Part model, mm, in its own coordinate system. Face numbers are marked on the shaded views. A direction names the side the tool comes from. Round coordinates to 2 decimals unless told otherwise and drop trailing zeros. Order: outer loops, then holes, each group sorted by start corner. A loop starts at its lowest first (then second) coordinate and runs counter-clockwise, first axis right, second up. Notation, with made-up numbers: M -33,2.25 L 25,2.25 A26 cw 25,38.25 Z; hole C 8.5,35.25 d9. An arc over 180 degrees is marked long. Write each question's results on one line, items separated by ' | '. Start each with the question number.
1. Two-plate mould, pull along Y, no slides. Class the marked faces 3, 4 and 5: +Y half, -Y half, draft (parallel to the pull), parting line (faces both ways), or undercut.
2. Drop flat-ended pins along their axis: pin 1 Ø1.6 at (x, z) = (45, -8.5) entering from -Y; pin 2 Ø4 at (y, z) = (7.5, 36) entering from -X; pin 3 Ø4 at (x, y) = (38.5, -9.5) entering from +Z. Give the stop position or say it passes through.
3. Probe L1, parallel to Y at x = 5, z = 38; L2, parallel to X at y = 2.25, z = -20; L3, parallel to Z at x = 25, y = 9.5. List the from-to ranges inside material, lowest first. Write a range as [from, to].
4. Band-saw the part on C-C, the plane y = -3.5. List the corners of the cut face in (x, z).
5. Band-saw the part on B-B, the plane y = 1.25. List the corners of the cut face in (x, z), then the cut area to 3 significant figures.
6. Which spindle directions (+Z, -Z, +X, -X, +Y, -Y) get a long thin tool onto all of the face, cutting with end or side? Do the marked faces 1 and 2. Say none if no direction does.
7. Band-saw the part on A-A, the plane z = 29.5. List the corners of the cut face in (x, y).
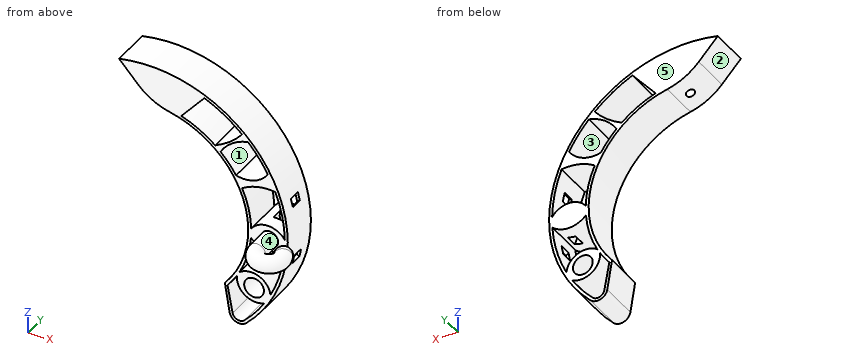
```python
from build123d import *

# Parameters (mm, degrees)
BOSS_EXTRUDE1_DEPTH        = 13.33
FILLET1_R                  = 20
SKETCH3_R                  = 3.33
CUT_EXTRUDE2_DEPTH         = 68.320131462
FILLET2_R                  = 3.333
SKETCH4_R                  = 2.8333333
DOME1_FACE_RADIUS          = 2.8333333
DOME1_HEIGHT               = 3.3333333
CUT_EXTRUDE3_DEPTH         = 2
MIRROR3_COPY_1_FACE_RADIUS = 2.8333333
MIRROR3_COPY_1_HEIGHT      = 3.3333333
SKETCH16_W                 = 36.728720905
SKETCH16_H                 = 19.011400322
CUT_EXTRUDE4_DEPTH         = 30
CUT_EXTRUDE5_DEPTH         = 71.999747127
SKETCH19_R                 = 1.425
CUT_EXTRUDE6_DEPTH         = 8.6


with BuildPart() as part:
    # Sketch1 → Boss-Extrude1 (new body)
    with BuildSketch(Plane(origin=(0, 0, 0), x_dir=(1, 0, 0), z_dir=(0, 1, 0))):
        with BuildLine():
            Line((25.438564969, 21.535280641), (27.993333135, 37.33))
            ThreePointArc((27.993333135, 37.33), (42.371570445, -19.53984693), (-10.216878485, -45.527694802))
            Line((-10.216878485, -45.527694802), (1.110949751, -33.311479863))
            ThreePointArc((1.110949751, -33.311479863), (30.46737546, -13.513990254), (25.438564969, 21.535280641))
        make_face()
    extrude(amount=BOSS_EXTRUDE1_DEPTH)

    # Fillet1
    fillet1_edges = [part.edges().sort_by_distance(p)[0] for p in [
        (1.110949751, 6.665, 33.311479863),
    ]]
    fillet(fillet1_edges, radius=FILLET1_R)

    # Sketch3 → Cut-Extrude2 (cut, through all)
    with BuildSketch(Plane(origin=(0, 13.33, 0), x_dir=(1, 0, 0), z_dir=(0, 1, 0))):
        with Locations(Location((35.289122258, 19.812921474, 0), (0, 0, 270))):
            Circle(SKETCH3_R)
    extrude(amount=-CUT_EXTRUDE2_DEPTH, mode=Mode.SUBTRACT)

    # Fillet2
    fillet2_edges = [part.edges().sort_by_distance(p)[0] for p in [
        (27.993333135, 6.665, -37.33),
    ]]
    fillet(fillet2_edges, radius=FILLET2_R)

    # Sweep1: sweep along a path in Sketch6
    with BuildLine(Plane.XY) as sweep1_path:
        Line((40.567020893, 13.33), (40.567020893, 20.636666))
        ThreePointArc((40.567020893, 20.636666), (45.529478945, 24.636666), (48.384610469, 18.938050913))
    # Sketch4 → Sweep1 (sweep)
    with BuildSketch(Plane(origin=(0, 13.33, 0), x_dir=(1, 0, 0), z_dir=(0, 1, 0))):
        with Locations((40.567020893, 0.715488074)):
            Circle(SKETCH4_R)
    sweep1 = sweep(path=sweep1_path.line)

    # Dome1: a dome of height H over a round flat face of radius A is a cap of a sphere of radius (A * A + H * H) / (2 * H)
    dome1_r = (DOME1_FACE_RADIUS * DOME1_FACE_RADIUS + DOME1_HEIGHT * DOME1_HEIGHT) / (2 * DOME1_HEIGHT)
    dome1_base = Plane((48.384610469, 18.938050913, -0.715488074), z_dir=(-0.414971112372, -0.909834587107, 0))
    with Locations(dome1_base.offset(DOME1_HEIGHT - dome1_r)):
        dome1_ball = Sphere(dome1_r, mode=Mode.PRIVATE)
    add(split(dome1_ball, bisect_by=dome1_base, keep=Keep.TOP, mode=Mode.PRIVATE))

    # Sketch7 → Cut-Extrude3 (cut, symmetric)
    with BuildSketch(Plane(origin=(0, 6.665, 0), x_dir=(1, 0, 0), z_dir=(0, 1, 0))):
        with BuildLine():
            ThreePointArc((44.965852541, -12.459041105), (45.327303444, -11.072089345), (45.645985213, -9.674690379))
            ThreePointArc((45.645985213, -9.674690379), (41.52914689, -0.997602982), (46.057874066, 7.47180276))
            ThreePointArc((46.057874066, 7.47180276), (45.806657105, 8.882891694), (45.51221871, 10.285599066))
            ThreePointArc((45.51221871, 10.285599066), (38.862616133, -0.933548234), (44.965852541, -12.459041105))
        make_face()
    extrude(amount=CUT_EXTRUDE3_DEPTH, both=True, mode=Mode.SUBTRACT)

    # Mirror3: Sweep1 across plane
    add(sweep1.mirror(Plane.ZX.offset(6.665)))

    # Mirror3 copy 1: a dome of height H over a round flat face of radius A is a cap of a sphere of radius (A * A + H * H) / (2 * H)
    mirror3_copy_1_r = (MIRROR3_COPY_1_FACE_RADIUS * MIRROR3_COPY_1_FACE_RADIUS + MIRROR3_COPY_1_HEIGHT * MIRROR3_COPY_1_HEIGHT) / (2 * MIRROR3_COPY_1_HEIGHT)
    mirror3_copy_1_base = Plane((48.384610469, -5.608050913, -0.715488074), z_dir=(-0.414971112372, 0.909834587107, 0))
    with Locations(mirror3_copy_1_base.offset(MIRROR3_COPY_1_HEIGHT - mirror3_copy_1_r)):
        mirror3_copy_1_ball = Sphere(mirror3_copy_1_r, mode=Mode.PRIVATE)
    add(split(mirror3_copy_1_ball, bisect_by=mirror3_copy_1_base, keep=Keep.TOP, mode=Mode.PRIVATE))

    # Sketch16 → Cut-Extrude4 (cut)
    with BuildSketch(Plane(origin=(0, 13.33, 0), x_dir=(1, 0, 0), z_dir=(0, 1, 0))):
        with Locations((41.954103887, 0)):
            Rectangle(SKETCH16_W, SKETCH16_H)
    extrude(amount=CUT_EXTRUDE4_DEPTH, mode=Mode.SUBTRACT)

    # Sketch18 → Cut-Extrude5 (cut, through all)
    with BuildSketch(Plane.XZ):
        with BuildLine():
            Line((28.039143401, -31.35294351), (26.341104847, -22.015791956))
            ThreePointArc((26.341104847, -22.015791956), (28.034108775, -19.815086303), (29.543730196, -17.484762112))
            ThreePointArc((29.543730196, -17.484762112), (32.195597251, -23.521489799), (38.760601016, -24.1340301))
            ThreePointArc((38.760601016, -24.1340301), (35.637384762, -28.544919116), (32.014856699, -32.555868143))
            ThreePointArc((32.014856699, -32.555868143), (29.659442281, -33.169198731), (28.039143401, -31.35294351))
        make_face()
        with BuildLine():
            Line((18.550254331, 41.721980589), (10.749078367, 32.603776074))
            ThreePointArc((10.749078367, 32.603776074), (16.777611199, 29.950970977), (22.188585816, 26.195716434))
            ThreePointArc((22.188585816, 26.195716434), (27.124492616, 29.226219474), (31.260994101, 33.280412374))
            ThreePointArc((31.260994101, 33.280412374), (25.260742984, 38.035910189), (18.550254331, 41.721980589))
        make_face()
        with BuildLine():
            ThreePointArc((40.820629514, -20.457561098), (36.928571374, -15.146521153), (30.394540812, -15.959974588))
            ThreePointArc((30.394540812, -15.959974588), (33.016991898, -9.403570916), (34.242514373, -2.449307946))
            ThreePointArc((34.242514373, -2.449307946), (39.834796056, -4.973265496), (45.573843855, -2.803632696))
            ThreePointArc((45.573843855, -2.803632696), (44.089869065, -11.870932812), (40.820629514, -20.457561098))
        make_face()
        with BuildLine():
            ThreePointArc((45.651589838, 0.876324867), (39.98520163, 3.873028579), (34.318813422, 0.876324867))
            ThreePointArc((34.318813422, 0.876324867), (33.458600037, 7.685764997), (31.260994101, 14.187993085))
            ThreePointArc((31.260994101, 14.187993085), (36.627069292, 16.498940097), (42.462553984, 16.785919968))
            ThreePointArc((42.462553984, 16.785919968), (44.769458221, 8.973918351), (45.651589838, 0.876324867))
        make_face()
        with BuildLine():
            ThreePointArc((39.931059829, 22.143758962), (35.264351947, 18.298272838), (29.224062449, 18.013968857))
            ThreePointArc((29.224062449, 18.013968857), (26.794540492, 21.461628545), (23.960583625, 24.58534792))
            ThreePointArc((23.960583625, 24.58534792), (27.897400776, 28.917406773), (33.24466644, 31.299005627))
            ThreePointArc((33.24466644, 31.299005627), (36.873111669, 26.929709168), (39.931059829, 22.143758962))
        make_face()
    extrude(amount=-CUT_EXTRUDE5_DEPTH, mode=Mode.SUBTRACT)

    # Sketch19 → Cut-Extrude6 (cut, symmetric)
    with BuildSketch(Plane(origin=(15.613362891, 0, 27.64706404), x_dir=(0.8707413871359999, 0, -0.491741229437267), z_dir=(0.491741229437267, 0, 0.8707413871359999))):
        with Locations(Location((-14.136648815, 6.665, 0), (0, 0, 180))):
            Circle(SKETCH19_R)
    extrude(amount=CUT_EXTRUDE6_DEPTH, both=True, mode=Mode.SUBTRACT)


solid = part.part
```
Solution:
1) face 3: draft | face 4: undercut | face 5: +Y half
2) pin 1: y = 0 | pin 2: x = -3.21 | pin 3: z = 2.08
3) L1: [0, 5.25], [8.08, 13.33] | L2: [26.66, 27.9], [29.74, 31.96], [38.61, 40.76], [41.05, 42.16] | L3: [22.04, 23.53], [26.12, 27.73], [38.21, 39.4]
4) outline: C 40.57,-0.72 d5.67; C 48.19,-0.72 d4.65
5) outline: M -10.22,45.53 L -3.81,38.61 A20 ccw 6.79,32.63 A33.33 cw 25.44,-21.54 L 27.05,-31.47 A3.33 ccw 32.67,-33.32 A46.66 ccw Z; hole M 10.75,32.6 A34.33 cw 22.19,26.2 A25.83 ccw 31.26,33.28 A45.66 ccw 18.55,41.72 Z; hole M 23.96,24.59 A34.33 cw 29.22,18.01 A9.58 ccw 39.93,22.14 A45.66 ccw 33.24,31.3 A14.24 ccw Z; hole M 26.34,-22.02 L 28.04,-31.35 A2.33 ccw 32.01,-32.56 A45.66 ccw 38.76,-24.13 A6.5 cw 29.54,-17.48 A34.33 cw Z; hole M 30.39,-15.96 A6.5 cw 40.82,-20.46 A45.66 ccw 45.57,-2.8 A8.02 cw 34.24,-2.45 A34.33 cw Z; hole M 31.26,14.19 A34.33 cw 34.32,0.88 A6.86 cw 45.65,0.88 A45.66 ccw 42.46,16.79 A16.43 ccw Z; hole C 35.29,-19.81 d6.66 | area: 615 mm^2
6) face 1: +Y, -Y | face 2: -Z, -X, +Y, -Y
7) outline: M 15.51,0 L 17.56,0 L 17.56,13.33 L 15.51,13.33 Z; M 27.47,0 L 28.77,0 L 28.77,13.33 L 27.47,13.33 Z; M 34.85,0 L 36.15,0 L 36.15,13.33 L 34.85,13.33 Z
